The model under review builds one solid part; all positions refer to its coordinate system, in mm. Give positions to 0.01 mm unless a question says otherwise; leave off trailing zeros. Order: outer loops, then holes, each group sorted by start corner. A loop starts at its lowest first (then second) coordinate and runs counter-clockwise, first axis right, second up. Notation, with made-up numbers: (57, 23.5) - (87, 23.5) arc R15 cw to (87, 37.5) - close; hole circle Ø11 at (50.25, -27.75). An arc over 180 degrees is marked (long way). Put each result on its own line as item: value.
Autodesk Inventor part; units mm, degrees
ref_plane "YZ Plane" through (0, 0, 0) normal (1, 0, 0) x (0, 1, 0)
ref_plane "XZ Plane" through (0, 0, 0) normal (0, 1, 0) x (-1, 0, 0)
ref_plane "XY Plane" through (0, 0, 0) normal (0, 0, 1) x (1, 0, 0)
sketch "Block1" plane through (0, 0, 0) normal (0, 0, 1) x (1, 0, 0)
  line L0 (0.22, -250.22) -> (-180.22, -250.22)
  line L1 (-180.22, -250.22) -> (-180.22, 0.22)
  line L2 (-180.22, 0.22) -> (0.22, 0.22)
  line L3 (0.22, 0.22) -> (0.22, -250.22)
  circle A0 centre (-10, -230) radius 2.72
  circle A1 centre (-10, -20) radius 2.72
  circle A2 centre (-170, -20) radius 2.72
  circle A3 centre (-170, -230) radius 2.72
  point P0 (-90, -125)
sketch "Sketch1" plane through (0, 0, 0) normal (0, 1, 0) x (-1, 0, 0)
  line L0 (0, 0) -> (180, 0)
  line L1 (180, 0) -> (180, 250)
  line L2 (180, 250) -> (0, 250)
  line L3 (0, 250) -> (0, 0)
  circle A0 centre (170, 230) radius 2.5
  line L4 (90, 267.688) -> (90, -13.7422)
  line L5 (215.5014, 125) -> (-35.5429, 125)
  circle A1 centre (10, 230) radius 2.5
  circle A2 centre (170, 20) radius 2.5
  circle A3 centre (10, 20) radius 2.5
  dimension "d1" = 250
  dimension "d2" = 180
  dimension "d5" = 5
  dimension "d6" = 10
  dimension "d7" = 20
  dimension "d8" = 90
  dimension "d9" = 125
extrude "Extrusion2" add sketch "Sketch1" along normal blind 10
sketch "Sketch2" plane through (0, 10, 0) normal (0, 1, 0) x (1, 0, 0)
  circle A0 centre (-10, -20) radius 2.5
  circle A1 centre (-170, -20) radius 2.5
  circle A2 centre (-10, -230) radius 2.5
  circle A3 centre (-170, -230) radius 2.5
  line L0 (0, 0) -> (-180, 0)
  line L1 (-180, 0) -> (-180, -250)
  line L2 (-180, -250) -> (0, -250)
  line L3 (0, -250) -> (0, 0)
sketch "DXF" plane through (0, 0, 0) normal (0, 1, 0) x (-1, 0, 0)
  point P0 (0, 0)
properties part number "guardplate"
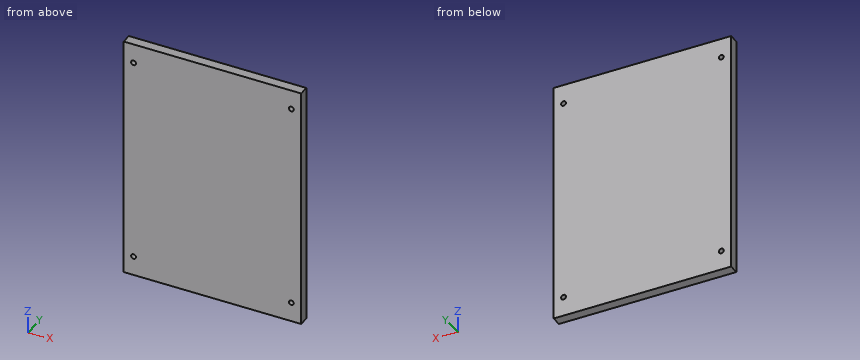
(1) Wall thickness on L1, parallel to X at y = 4.5, z = 230; L2, parallel to Z at x = -10, y = 4; L3, parallel to Z at x = -168, y = 3.75: over which ranges is each line inside the solid? List them lowest first.
The answers:
L1: -180 to -172.5, -167.5 to -12.5, -7.5 to 0
L2: 0 to 17.5, 22.5 to 227.5, 232.5 to 250
L3: 0 to 18.5, 21.5 to 228.5, 231.5 to 250
(2) Take a section at A-A, the plane x = -170. Write out the cut boundary in (y, z).
The answers:
outline: (0, 0) - (10, 0) - (10, 17.5) - (0, 17.5) - close; (0, 22.5) - (10, 22.5) - (10, 227.5) - (0, 227.5) - close; (0, 232.5) - (10, 232.5) - (10, 250) - (0, 250) - close
(3) Take a section at B-B, the plane z = 230. Write out the cut boundary in (x, y), then the cut area to 3 significant figures.
The answers:
outline: (-180, 0) - (-172.5, 0) - (-172.5, 10) - (-180, 10) - close; (-167.5, 0) - (-12.5, 0) - (-12.5, 10) - (-167.5, 10) - close; (-7.5, 0) - (0, 0) - (0, 10) - (-7.5, 10) - close
area: 1,700 mm^2
